```python
from build123d import *

# Parameters (mm, degrees)
BASE_WALLS_DEPTH     = 72
BOX_SHELL_T          = -5
SHAFT_HOLE_PROFILE_R = 3.5
CUT_EXTRUDE1_DEPTH   = 129.195163715


with BuildPart() as part:
    # Base Top Face Profile → Base Walls (new body)
    with BuildSketch(Plane(origin=(0, 0, 0), x_dir=(1, 0, 0), z_dir=(0, 1, 0))):
        with BuildLine():
            Line((-55, -75), (55, -75))
            ThreePointArc((55, -75), (69.142135624, -69.142135624), (75, -55))
            Line((75, -55), (75, 55))
            ThreePointArc((75, 55), (69.142135624, 69.142135624), (55, 75))
            Line((55, 75), (-55, 75))
            ThreePointArc((-55, 75), (-69.142135624, 69.142135624), (-75, 55))
            Line((-75, 55), (-75, -55))
            ThreePointArc((-75, -55), (-69.142135624, -69.142135624), (-55, -75))
        make_face()
    extrude(amount=-BASE_WALLS_DEPTH)

    # Box Shell
    box_shell_openings = [part.faces().sort_by_distance(p)[0] for p in [
        (0, -72, 0),
    ]]
    offset(amount=BOX_SHELL_T, openings=box_shell_openings, kind=Kind.INTERSECTION)

    # Shaft Hole Profile → Cut-Extrude1 (cut, through all)
    with BuildSketch(Plane(origin=(0, 0, 0), x_dir=(1, 0, 0), z_dir=(0, 1, 0))):
        with Locations(Location((0, 0, 0), (0, 0, 270))):
            Circle(SHAFT_HOLE_PROFILE_R)
    extrude(amount=-CUT_EXTRUDE1_DEPTH, mode=Mode.SUBTRACT)


solid = part.part
```
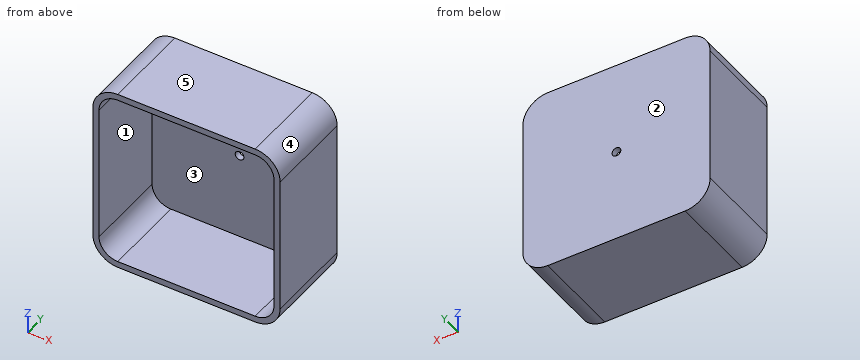
For this review, take the finished solid that the model builds, in its own axes (mm). Face numbers are marked on the shaded views. A direction names the side the tool comes from. Coordinates: 2 decimals unless noted, no trailing zeros. Loops run counter-clockwise (first coordinate to the right, second up) from the corner with the lowest first, then second, coordinate; pieces in that order, holes last. Notation, with made-up numbers: (-8, 5) - (36, 5) arc R20 cw to (36, 30) - close; hole circle Ø7 at (-3, 68). An arc over 180 degrees is marked (long way). Use one line per item in the form item = value. Start each with the question number.
1) Take a section at A-A (x = 0). State the section outline as (y, z) points.
2) Draft analysis for pull direction X (two halves, no side actions). For the marked faces 3, 4 and 5, state which applies: released by +X, released by -X, zero draft, split by the parting line, or undercut.
3) Take a section at B-B (y = -14.5). State the section outline as (x, z) points.
4) Take a section at D-D (x = -23.5). State the section outline as (y, z) points, plus the area to 3 significant figures.
5) To check wall thickness, follow probe 1 along Z at (x, y) = (35, -41); probe 2 along X at (y, z) = (-2.35, 0). State the ranges of each line that lie inside material, in increasing order. Write a range as from..to.
6) Take a section at C-C (z = 0). State the section outline as (x, y) points.
7) For the marked faces 1 and 2, list the 3-axis set-ups (+Z, -Z, +X, -X, +Y, -Y) from which the entire face can be reached by the end or side of a thin tool; tool diameter is ignored.
8) For pin 1 (8 mm diameter, centred on x = 0, z = 0, fed in from -Y); pin 2 (3 mm diameter, centred on y = -45, z = 57.5, fed in from +X) (3 decimals), all flat-tipped, find the tip position at first contact; note any pin that passes through.
From the geometry:
q1.outline = (-72, -75) - (0, -75) - (0, -3.5) - (-5, -3.5) - (-5, -70) - (-72, -70) - close; (-72, 70) - (-5, 70) - (-5, 3.5) - (0, 3.5) - (0, 75) - (-72, 75) - close
q2.face_3 = undercut
q2.face_4 = released by +X
q2.face_5 = zero draft
q3.outline = (-75, -55) arc R20 ccw to (-55, -75) - (55, -75) arc R20 ccw to (75, -55) - (75, 55) arc R20 ccw to (55, 75) - (-55, 75) arc R20 ccw to (-75, 55) - close; hole (-70, -55) arc R15 ccw to (-55, -70) - (55, -70) arc R15 ccw to (70, -55) - (70, 55) arc R15 ccw to (55, 70) - (-55, 70) arc R15 ccw to (-70, 55) - close
q4.outline = (-72, -75) - (0, -75) - (0, 75) - (-72, 75) - (-72, 70) - (-5, 70) - (-5, -70) - (-72, -70) - close
q4.area = 1,420 mm2
q5.probe_1 = -75..-70, 70..75
q5.probe_2 = -75..-3.5, 3.5..75
q6.outline = (-75, -72) - (-70, -72) - (-70, -5) - (-3.5, -5) - (-3.5, 0) - (-75, 0) - close; (3.5, -5) - (70, -5) - (70, -72) - (75, -72) - (75, 0) - (3.5, 0) - close
q7.face_1 = -Y
q7.face_2 = +Z, -Z, +X, -X, +Y
q8.pin_1 = -5
q8.pin_2 = 74.975
